Here's how the part is built. I have some questions about the finished solid (model axes, mm). Face numbers are marked on the shaded views. Round coordinates to 2 decimals unless told otherwise and drop trailing zeros. Loops run counter-clockwise (first coordinate to the right, second up) from the corner with the lowest first, then second, coordinate; pieces in that order, holes last. Notation, with made-up numbers: M 11.5,14.25 L 63.5,14.25 A11 cw 63.5,19.25 Z; hole C 8,77.5 d3. An arc over 180 degrees is marked long. Use a Markdown table: item, result.
Autodesk Fusion 360 part; units mm, degrees
sketch "Sketch1" plane through (0, 0, 0) normal (0, 0, 1) x (1, 0, 0)
  line L0 (21.25, 21.25) -> (-21.25, 21.25)
  line L1 (-21.25, 21.25) -> (-21.25, -21.25)
  line L2 (-21.25, -21.25) -> (21.25, -21.25)
  line L3 (21.25, -21.25) -> (21.25, 21.25)
  line L4 (21.25, 21.25) -> (-21.25, -21.25) construction
  line L5 (-21.25, 21.25) -> (21.25, -21.25) construction
  line L6 (25.25, -25.25) -> (-25.25, -25.25)
  line L7 (-25.25, -25.25) -> (-25.25, 25.25)
  line L8 (-25.25, 25.25) -> (25.25, 25.25)
  line L9 (25.25, 25.25) -> (25.25, -25.25)
  line L10 (25.25, -25.25) -> (-25.25, 25.25) construction
  line L11 (-25.25, -25.25) -> (25.25, 25.25) construction
  line L12 (-21.25, 0) -> (-25.25, 0)
  dimension "d2" = 42.5
  dimension "d3" = 42.5
  dimension "d4" = 4
extrude "Extrude1" add sketch "Sketch1" along normal blind 3.2
sketch "Sketch2" plane through (0, 0, 0) normal (0, 0, 1) x (1, 0, 0)
  circle A0 centre (0, 0) radius 40.4366
  circle A1 centre (0, 0) radius 45.4366
  line L0 (0.1635, 40.4363) -> (0.1635, 45.4363)
  dimension "d7" = 5
extrude "Extrude2" add sketch "Sketch2" against normal blind 5 contours A0 | A1
sketch "Sketch3" plane through (0, 0, 0) normal (0, 0, 1) x (1, 0, 0)
sketch "Sketch4" plane through (0, 0, 0) normal (0, 0, 1) x (1, 0, 0)
  line L0 (25.25, 25.25) -> (25.25, -25.25)
  line L1 (25.25, -25.25) -> (-25.25, -25.25)
  line L2 (-25.25, -25.25) -> (-25.25, 25.25)
  line L3 (-25.25, 25.25) -> (25.25, 25.25)
  circle A0 centre (0, 0) radius 45.4366
  circle A1 centre (0, 33.5) radius 5.5
extrude "Extrude3" cut sketch "Sketch4" against normal blind 10 contours A1
sketch "Sketch5" plane through (0, 0, 0) normal (0, 0, 1) x (1, 0, 0)
extrude "Extrude4" add sketch "Sketch2" along normal blind 64.5
sketch "Sketch6" plane through (0, 0, 0) normal (0, 0, 1) x (1, 0, 0)
  point P0 (-45.4366, 0)
ref_plane "WorkPlane1" through (0, 0, 64.5) normal (0, 0, 1) x (1, 0, 0)
sketch "Sketch7" plane through (0, 0, 64.5) normal (0, 0, 1) x (1, 0, 0)
  line L0 (-6.3568, -39.7886) -> (6.6432, -39.7886)
  line L1 (6.6432, -39.7886) -> (6.6432, -45.6886)
  line L2 (6.6432, -45.6886) -> (-6.3568, -45.6886)
  line L3 (-6.3568, -45.6886) -> (-6.3568, -39.7886)
  dimension "d15" = 5.9
  dimension "d16" = 13
extrude "Extrude5" cut sketch "Sketch7" against normal blind 6
sketch "Sketch8" plane through (0, 0, 0) normal (1, 0, 0) x (0, 1, 0)
  line L0 (-45.4366, 58.5) -> (-45.4366, -5)
  line L1 (45.4366, -5) -> (45.4366, 64.5)
  line L2 (0, 64.5) -> (0, -5) construction
  line L3 (-5.5, 34.75) -> (5.5, 34.75)
  line L4 (5.5, 34.75) -> (5.5, 29.75)
  line L5 (5.5, 29.75) -> (-5.5, 29.75)
  line L6 (-5.5, 29.75) -> (-5.5, 34.75)
  line L7 (45.4366, 64.5) -> (-44.9897, 64.5)
  line L8 (-45.4366, -5) -> (45.4366, -5)
  dimension "d19" = 11
  dimension "d20" = 5
extrude "Extrude6" cut sketch "Sketch8" along normal mid plane 200
sketch "Sketch9" plane through (0, 0, 0) normal (1, 0, 0) x (0, 1, 0)
  line L0 (-8.5, 36.25) -> (8.5, 36.25)
  line L1 (8.5, 36.25) -> (8.5, 23.25)
  line L2 (8.5, 23.25) -> (-8.5, 23.25)
  line L3 (-8.5, 23.25) -> (-8.5, 36.25)
  line L4 (0, 64.5) -> (0, -5)
  line L5 (-45.4366, -5) -> (45.4366, -5)
  line L6 (45.4366, 64.5) -> (-44.9897, 64.5)
  line L7 (0, 36.25) -> (0, 23.25)
  dimension "d23" = 17
  dimension "d24" = 13
extrude "Extrude7" cut sketch "Sketch9" along normal mid plane 84
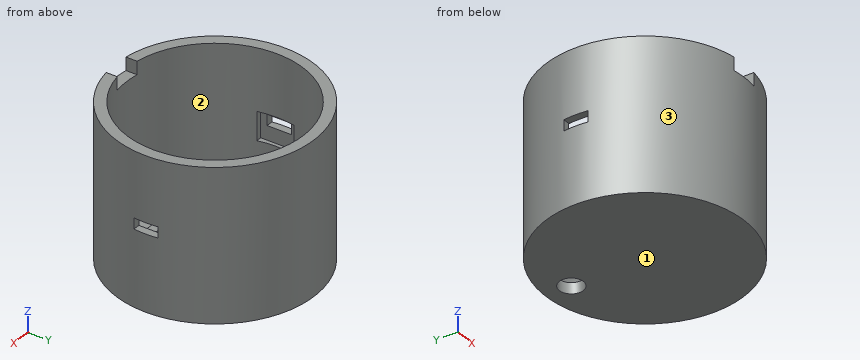
1. For pin 1 Ø8 at (y, z) = (3, 3.5) entering from +X; pin 2 Ø6 at (x, y) = (2, -43.5) entering from +Z; pin 3 Ø8 at (y, z) = (-32.5, 11.5) entering from -X; pin 4 Ø3 at (y, z) = (-4.5, 54.5) entering from +X, each with a flat end and sliding along its axis, tell me the tip position at first contact or that it passes through.
Answer sheet:
| item | result |
|---|---|
| pin 1 | x = 45.44 |
| pin 2 | z = 58.5 |
| pin 3 | x = -35.39 |
| pin 4 | x = 45.34 |
2. Imagine slicing it at B-B, the plane z = 31.5. Write out the boundary of the cut face in (x, y).
Answer sheet:
| item | result |
|---|---|
| outline | M -45.1,-5.5 A45.44 ccw 45.1,-5.5 L 42,-5.5 L 42,-8.5 L 39.53,-8.5 A40.44 cw -39.53,-8.5 L -42,-8.5 L -42,-5.5 Z; M -45.1,5.5 L -42,5.5 L -42,8.5 L -39.53,8.5 A40.44 cw 39.53,8.5 L 42,8.5 L 42,5.5 L 45.1,5.5 A45.44 ccw Z |
3. I need wall thicknesses on probe 1 along Y at (x, z) = (0, -1.95); probe 2 along X at (y, z) = (0, 48.5); probe 3 along Z at (x, y) = (-7.5, 26). Which ranges of each line are inside material? Lowest first, please. Write a range as from..to.
Answer sheet:
| item | result |
|---|---|
| probe 1 | -45.44..28, 39..45.44 |
| probe 2 | -45.44..-40.44, 40.44..45.44 |
| probe 3 | -5..0 |
4. Imagine slicing it at A-A, the plane y = 0. State how many separate pieces and enclosed holes the cut face has, then the cut area to 3 significant figures.
Answer sheet:
| item | result |
|---|---|
| separate pieces | 3 |
| enclosed holes | 0 |
| area | 1,050 mm2 |
5. Imagine slicing it at C-C, the plane x = 0. Write out the boundary of the cut face in (y, z), then the cut area to 3 significant figures.
Answer sheet:
| item | result |
|---|---|
| outline | M -45.44,-5 L 28,-5 L 28,0 L 25.25,0 L 25.25,3.2 L 21.25,3.2 L 21.25,0 L -21.25,0 L -21.25,3.2 L -25.25,3.2 L -25.25,0 L -40.44,0 L -40.44,58.5 L -45.44,58.5 Z; M 39,-5 L 45.44,-5 L 45.44,64.5 L 40.44,64.5 L 40.44,0 L 39,0 Z |
| area | 1,040 mm2 |
6. Imagine slicing it at D-D, the plane z = 20. Write out the boundary of the cut face in (x, y), then the cut area to 3 significant figures.
Answer sheet:
| item | result |
|---|---|
| outline | C 0,0 d90.87; hole C 0,0 d80.87 |
| area | 1,350 mm2 |
7. We'd pull the mould along Y, two halves only. Please class the marked faces 1, 2 and 3: +Y half, -Y half, draft (parallel to the pull), parting line (faces both ways), or undercut.
Answer sheet:
| item | result |
|---|---|
| face 1 | draft |
| face 2 | undercut |
| face 3 | parting line |
